For this review, take the finished solid that the model builds, in its own axes (mm). Round coordinates to 2 decimals unless told otherwise and drop trailing zeros. Loops run counter-clockwise (first coordinate to the right, second up) from the corner with the lowest first, then second, coordinate; pieces in that order, holes last.
1. Draft analysis for pull direction Y (two halves, no side actions). For faces 1 (the cylindrical face through (34.83, -217.39, -1.51)), 2 (the flat face through (1, -220, -14)), 3 (the flat face through (38, -206, -1)), state which applies: released by +Y, released by -Y, zero draft, split by the parting line, or undercut.
2. Consider section A-A on y = -198.5. State the section outline as (x, z) points.
3. Consider section C-C on x = 6.5. State the section outline as (y, z) points.
4. Consider section D-D on x = -15.5. State the section outline as (y, z) points.
5. Clearance check with flat-ended pins moving along their axes: pin 1 Ø8 at (x, z) = (24.5, -14.5) entering from +Y; pin 2 Ø4 at (x, z) = (34.64, -24.84) entering from -Y; pin 3 Ø1.9 at (x, y) = (34.57, -186.03) entering from +Z; pin 4 Ø3 at (x, y) = (34.57, -216.22) entering from -Z. State where each tip first meets the part, or that it passes through.
6. Consider section B-B on z = -6. State the section outline as (x, y) points.
7. To check wall thickness, follow line 1 along Z through (x, y) = (-11, -187.5); line 2 along Y through (x, z) = (-33, -8.5); line 3 along Y through (x, z) = (32, -1.75). State the ranges of each line that lie inside material, in increasing order.
from build123d import *

# Parameters (mm, degrees)
BOSS_EXTRUDE1_DEPTH                                 = 2
SKETCH2_W                                           = 76
SKETCH2_H                                           = 2
BOSS_EXTRUDE2_DEPTH                                 = 26
CSK_FOR_M2_COUNTERSUNK_FLAT_HEAD_SCREW1_D           = 2.4
CSK_FOR_M2_COUNTERSUNK_FLAT_HEAD_SCREW1_CSINK_D     = 4.4
CSK_FOR_M2_COUNTERSUNK_FLAT_HEAD_SCREW1_CSINK_ANGLE = 90
CSK_FOR_M2_COUNTERSUNK_FLAT_HEAD_SCREW2_D           = 2.4
CSK_FOR_M2_COUNTERSUNK_FLAT_HEAD_SCREW2_CSINK_D     = 4.4
CSK_FOR_M2_COUNTERSUNK_FLAT_HEAD_SCREW2_CSINK_ANGLE = 90


with BuildPart() as part:
    # Sketch1 → Boss-Extrude1 (new body)
    with BuildSketch(Plane.XY):
        with BuildLine():
            Line((38, -220), (38, -180.544315889))
            ThreePointArc((38, -180.544315889), (0, -184.5), (-38, -180.544315889))
            Line((-38, -180.544315889), (-38, -220))
            Line((-38, -220), (38, -220))
        make_face()
    extrude(amount=-BOSS_EXTRUDE1_DEPTH)

    # Sketch2 → Boss-Extrude2 (add)
    with BuildSketch(Plane(origin=(0, 0, -2), x_dir=(-1, 0, 0), z_dir=(0, 0, -1))):
        with Locations((0, -219)):
            Rectangle(SKETCH2_W, SKETCH2_H)
    extrude(amount=BOSS_EXTRUDE2_DEPTH)

    # CSK for M2 Countersunk Flat Head Screw1 (through all)
    with Locations(Plane.XY):
        with Locations((-35.5, -216.217638504), (-35.5, -185.148473071), (1.425070676, -188.349538601), (34.565513804, -186.027196942), (34.565513804, -216.217638504)):
            CounterSinkHole(CSK_FOR_M2_COUNTERSUNK_FLAT_HEAD_SCREW1_D / 2, CSK_FOR_M2_COUNTERSUNK_FLAT_HEAD_SCREW1_CSINK_D / 2, counter_sink_angle=CSK_FOR_M2_COUNTERSUNK_FLAT_HEAD_SCREW1_CSINK_ANGLE)

    # CSK for M2 Countersunk Flat Head Screw2 (through all)
    with Locations(Plane(origin=(0, -220, 0), x_dir=(-1, 0, 0), z_dir=(0, -1, 0))):
        with Locations((-34.643963319, 24.841526038), (0, 25.688115944), (32.966559476, 23.505132472)):
            CounterSinkHole(CSK_FOR_M2_COUNTERSUNK_FLAT_HEAD_SCREW2_D / 2, CSK_FOR_M2_COUNTERSUNK_FLAT_HEAD_SCREW2_CSINK_D / 2, counter_sink_angle=CSK_FOR_M2_COUNTERSUNK_FLAT_HEAD_SCREW2_CSINK_ANGLE)


solid = part.part
Resolved:
1. face 1: undercut
1. face 2: released by -Y
1. face 3: zero draft
2. outline: (-38, -2) - (38, -2) - (38, 0) - (-38, 0) - close
3. outline: (-220, -28) - (-218, -28) - (-218, -2) - (-184.39, -2) - (-184.39, 0) - (-220, 0) - close
4. outline: (-220, -28) - (-218, -28) - (-218, -2) - (-183.85, -2) - (-183.85, 0) - (-220, 0) - close
5. pin 1: stops at y = -218
5. pin 2: stops at y = -219.8
5. pin 3: passes through
5. pin 4: stops at z = -2
6. outline: (-38, -220) - (38, -220) - (38, -218) - (-38, -218) - close
7. line 1: z = -2 to 0
7. line 2: y = -220 to -218
7. line 3: y = -220 to -181.7
